The model under review builds one solid part; all positions refer to its coordinate system, in mm. Coordinates: 2 decimals unless noted, no trailing zeros. Write each loop counter-clockwise with the first axis right and the second up, starting at its lowest first coordinate (ties: lowest second). Pieces come first, ordered by that corner, then holes. Notation, with made-up numbers: (65, 63.25) - (85, 63.25) arc R24 ccw to (85, 97.25) - close; hole circle Ø11 at (60, 42). An arc over 180 degrees is marked (long way). Put each result on its own line as item: value.
from build123d import *

# Parameters (mm, degrees)
F0_W     = 508
F0_H     = 57.15
F1_DEPTH = 3.175
F4_DEPTH = 25.4
F2_W     = 101.6
F2_H     = 3.175
F5_DEPTH = 25.4
F6_W     = 101.6
F6_H     = 3.175
F7_DEPTH = 25.4


with BuildPart() as f1:
    # F0 (on Top) → F1 (new body)
    with BuildSketch(Plane.XY):
        with Locations((254, 28.575)):
            Rectangle(F0_W, F0_H)
    extrude(amount=F1_DEPTH)

    # F3 (on face) → F4 (cut)
    with BuildSketch(Plane.XY.offset(3.175)):
        Polygon((508, 50.8), (254, 0), (508, 0), align=None)
    extrude(amount=-F4_DEPTH, mode=Mode.SUBTRACT)

    # F2 (on face) → F5 (cut)
    with BuildSketch(Plane.XY.offset(3.175)):
        with Locations((50.8, 55.5625)):
            Rectangle(F2_W, F2_H)
        with Locations((254, 55.5625)):
            Rectangle(F2_W, F2_H)
        with Locations((457.2, 55.5625)):
            Rectangle(F2_W, F2_H)
    extrude(amount=-F5_DEPTH, mode=Mode.SUBTRACT)

    # F6 (on face) → F7 (cut)
    with BuildSketch(Plane.XY.offset(3.175)):
        with Locations((457.2, 52.3875)):
            Rectangle(F6_W, F6_H)
    extrude(amount=-F7_DEPTH, mode=Mode.SUBTRACT)


solid = f1.part
1. Consider section C-C on y = 34. State the section outline as (x, z) points (3 decimals).
Determined:
outline: (0, 0) - (424, 0) - (424, 3.175) - (0, 3.175) - close
2. To check wall thickness, follow probe 1 along Y at (x, z) = (28.5, 3) (3 decimals); probe 2 along X at (y, z) = (53, 0.45); probe 3 along Y at (x, z) = (483.5, 2.55). State the ranges of each line that lie inside material, in increasing order.
Determined:
probe 1: y = 0 to 53.975
probe 2: x = 0 to 406.4
probe 3: y = 45.9 to 50.8
3. Consider section B-B on x = 229. State the section outline as (y, z) points (3 decimals), plus the area to 3 significant figures.
Determined:
outline: (0, 0) - (53.975, 0) - (53.975, 3.175) - (0, 3.175) - close
area: 171 mm^2
4. Consider section A-A on z = 2.25. State the section outline as (x, y) points (3 decimals).
Determined:
outline: (0, 0) - (254, 0) - (508, 50.8) - (406.4, 50.8) - (406.4, 57.15) - (304.8, 57.15) - (304.8, 53.975) - (203.2, 53.975) - (203.2, 57.15) - (101.6, 57.15) - (101.6, 53.975) - (0, 53.975) - close
5. For pin 1 Ø1 at (y, z) = (55, 2.5) entering from +X; pin 2 Ø1.6 at (y, z) = (56, 2.5) entering from -X; pin 3 Ø1.5 at (x, z) = (311.5, 2) entering from -Y; pin 4 Ø1.5 at (x, y) = (429.5, 34) entering from +Z, all flat-tipped, find the tip position at first contact; note any pin that passes through.
Determined:
pin 1: stops at x = 406.4
pin 2: stops at x = 101.6
pin 3: stops at y = 11.35
pin 4: passes through
